Geometry: final body of the model. Coordinates: model frame, mm. A direction names the side the tool comes from. Round coordinates to 2 decimals unless told otherwise and drop trailing zeros. Loops run counter-clockwise (first coordinate to the right, second up) from the corner with the lowest first, then second, coordinate; pieces in that order, holes last. Notation, with made-up numbers: (70, 57) - (109, 57) arc R26 cw to (109, 79) - close; hole circle Ø5 at (59.5, -22). An arc over 180 degrees is marked (long way). Answer in a Markdown table with one row per item. Add a question column.
Autodesk Inventor part; units mm, degrees
ref_plane "YZ Plane" through (0, 0, 0) normal (1, 0, 0) x (0, 1, 0)
ref_plane "XZ Plane" through (0, 0, 0) normal (0, 1, 0) x (-1, 0, 0)
ref_plane "XY Plane" through (0, 0, 0) normal (0, 0, 1) x (1, 0, 0)
sketch "Sketch1" plane through (0, 0, 0) normal (0, 0, 1) x (1, 0, 0)
  line L0 (0, 0) -> (24, 0)
  line L1 (24, 0) -> (24, -60)
  line L2 (24, -60) -> (0, -60)
  line L3 (0, -60) -> (0, 0)
  dimension "d0" = 24
  dimension "d1" = 60
extrude "Extrusion1" add sketch "Sketch1" along normal blind 9
sketch "Sketch2" plane through (0, 0, 9) normal (0, 0, 1) x (1, 0, 0)
  line L0 (0, -60) -> (24, -60)
  line L1 (4, -55) -> (4, -10.95)
  line L2 (20, -10.95) -> (20, -55)
  line L3 (4, -10.95) -> (20, -10.95)
  line L4 (4, -55) -> (20, -55)
  line L5 (24, -60) -> (24, 0)
  line L6 (0, 0) -> (0, -60)
  line L7 (24, 0) -> (0, 0)
  dimension "d7" = 4
  dimension "d8" = 4
  dimension "d9" = 5
  dimension "d10" = 10.95
extrude "Extrusion2" cut sketch "Sketch2" against normal blind 5.5 contours L1 L3 L2 L4
sketch "Sketch3" plane through (24, -60, 0) normal (1, 0, 0) x (0, 0, -1)
  circle A0 centre (-1.5, 3) radius 0.5
  circle A1 centre (-1.5, 57) radius 0.5
  line L0 (0, 0) -> (-9, 0)
  line L1 (-9, 0) -> (-9, 60)
  line L2 (0, 60) -> (-9, 60)
  dimension "d15" = 1
  dimension "d18" = 1
  dimension "d19" = 3
  dimension "d20" = 7.5
  dimension "d21" = 3
  dimension "d22" = 7.5
extrude "Extrusion3" cut sketch "Sketch3" against normal blind 24
properties part number "Prueba1MPU"
1) Contact query for a flat-ended pin moving along its axis: pin 1 Ø3 at (x, y) = (17.5, -17.5) entering from +Z. Output: stop coordinate, or through.
2) Material intervals for line 1 along Y through (x, z) = (10.5, 1.5); line 2 along X through (y, z) = (-35.5, 4); line 3 along Z through (x, y) = (16.5, -57), sorted ascending. Write a range as from..to.
3) Reachability of faces 4 (the cylindrical face through (12, -3, 2)), 5 (the flat face through (12, -33, 3.5)) from +Z, -Z, +X, -X, +Y, -Y: full face, straight path, thin tool, end or side. Return the list, or none.
4) Pull-direction query (Y, two-part tool) for faces 1 (the flat face through (12, -30, 0)), 2 (the flat face through (4, -33, 6)), 3 (the flat face through (12, -60, 4)); classes: pulls with the +Y half, pulls with the -Y half, needs draft (parallel to the pull), parting line crosses it, or undercut.
5) Section B-B, the plane x = 10.25. Return the cut outline in (y, z), and give its area (3 significant figures).
6) Section C-C, the plane z = 6.25. Return the cut outline in (x, y).
7) Section A-A, the plane y = -40.5. Return the cut outline in (x, z).
Evaluation:
| question | item | result |
|---|---|---|
| 1 | pin 1 | stops at z = 3.5 |
| 2 | line 1 | y = -60..-57.5, -56.5..-3.5, -2.5..0 |
| 2 | line 2 | x = 0..4, 20..24 |
| 2 | line 3 | z = 0..1, 2..9 |
| 3 | face 4 | +X, -X |
| 3 | face 5 | +Z |
| 4 | face 1 | needs draft |
| 4 | face 2 | undercut |
| 4 | face 3 | pulls with the -Y half |
| 5 | outline | (-60, 0) - (0, 0) - (0, 9) - (-10.95, 9) - (-10.95, 3.5) - (-55, 3.5) - (-55, 9) - (-60, 9) - close; hole circle Ø1 at (-57, 1.5); hole circle Ø1 at (-3, 1.5) |
| 5 | area | 296 mm² |
| 6 | outline | (0, -60) - (24, -60) - (24, 0) - (0, 0) - close; hole (4, -55) - (20, -55) - (20, -10.95) - (4, -10.95) - close |
| 7 | outline | (0, 0) - (24, 0) - (24, 9) - (20, 9) - (20, 3.5) - (4, 3.5) - (4, 9) - (0, 9) - close |
